Could you check a few things on this model? Use its own coordinates, in mm. A direction names the side the tool comes from. Round coordinates to 2 decimals unless told otherwise and drop trailing zeros. Order: outer loops, then holes, each group sorted by start corner. A loop starts at its lowest first (then second) coordinate and runs counter-clockwise, first axis right, second up. Notation, with made-up numbers: (-17.75, 71) -> (41.25, 71) arc R19 ccw to (41.25, 90) -> close; hole circle Ø9 at (2.25, 44.25). An arc over 180 degrees is marked (long way). Put each result on its own line as item: value. Start each with the question number.
from build123d import *

# Parameters (mm, degrees)
BOSS_EXTRUDE1_DEPTH            = 1.14
F_3_2_3_2_DIAMETER_HOLE1_D     = 3.2
F_3_2_3_2_DIAMETER_HOLE1_DEPTH = 10
F_3_2_3_2_DIAMETER_HOLE1_TIP   = 0.96137699


with BuildPart() as part:
    # Sketch1 → Boss-Extrude1 (new body, symmetric)
    with BuildSketch(Plane(origin=(0, 0, 2279.99997139), x_dir=(1, 0, 0), z_dir=(0, 1, 0))):
        with BuildLine():
            Line((10, 2292.262711431), (10, 2309.99997139))
            Line((10, 2309.99997139), (0, 2309.99997139))
            Line((0, 2309.99997139), (0, 2279.99997139))
            Line((0, 2279.99997139), (20, 2279.99997139))
            Line((20, 2279.99997139), (20, 2289.99997139))
            Line((20, 2289.99997139), (12.262740041, 2289.99997139))
            ThreePointArc((12.262740041, 2289.99997139), (9.99862915, 2289.99860054), (10, 2292.262711431))
        make_face()
    extrude(amount=BOSS_EXTRUDE1_DEPTH, both=True)

    # Ø3.2 (3.2) Diameter Hole1
    with Locations(Plane(origin=(0, 1.14, 0), x_dir=(1, 0, 0), z_dir=(0, 1, 0))):
        with Locations((5, 25), (5, 5), (15, 5), (5, 15)):
            Hole(F_3_2_3_2_DIAMETER_HOLE1_D / 2, depth=F_3_2_3_2_DIAMETER_HOLE1_DEPTH)
            with Locations((0, 0, -(F_3_2_3_2_DIAMETER_HOLE1_DEPTH + F_3_2_3_2_DIAMETER_HOLE1_TIP / 2))):  # 118° drill point
                Cone(0, F_3_2_3_2_DIAMETER_HOLE1_D / 2, F_3_2_3_2_DIAMETER_HOLE1_TIP, mode=Mode.SUBTRACT)


solid = part.part
1. Thinking about a two-plate mould opening in Z: for faces 1 (the face through (5, 0, -30)), 2 (the face through (16.6, -0.02, -5.07)), 3 (the face through (10, 0, -21)), which applies, +Z half, -Z half, draft (parallel to the pull), parting line (faces both ways), or undercut?
2. If we section it at A-A, the plane x = 5: Please give me the cut outline in (y, z), then the cut area to 3 significant figures.
3. If we section it at D-D, the plane x = 15: Please give me the cut outline in (y, z), then the cut area to 3 significant figures.
4. I need wall thicknesses on L1, parallel to Z at x = 5, y = -0.6; L2, parallel to X at y = 0.05, z = -5; L3, parallel to X at y = -0.2, z = -15. Which ranges of each line are inside material? Lowest first, please.
5. If we section it at B-B, the plane y = -0.2: Please give me the cut outline in (x, z), then the cut area to 3 significant figures.
6. For pin 1 Ø0.7 at (y, z) = (0.5, -17.5) entering from +X; pin 2 Ø1 at (x, y) = (12, 0.5) entering from -Z, each with a flat end and sliding along its axis, tell me the tip position at first contact or that it passes through.
7. Which directions (+Z, -Z, +X, -X, +Y, -Y) give clear straight access to the entire face, cutting with the end or side of a thin tool? Please do faces 4 (the face through (8, 1.14, -12)), 5 (the face through (16, 0, -10)).
8. If we section it at C-C, the plane z = -5: Please give me the cut outline in (x, y), then the cut area to 3 significant figures.
Results below:
1. face 1: -Z half
1. face 2: undercut
1. face 3: draft
2. outline: (-1.14, -30) -> (1.14, -30) -> (1.14, -26.6) -> (-1.14, -26.6) -> close; (-1.14, -23.4) -> (1.14, -23.4) -> (1.14, -16.6) -> (-1.14, -16.6) -> close; (-1.14, -13.4) -> (1.14, -13.4) -> (1.14, -6.6) -> (-1.14, -6.6) -> close; (-1.14, -3.4) -> (1.14, -3.4) -> (1.14, 0) -> (-1.14, 0) -> close
2. area: 46.5 mm2
3. outline: (-1.14, -10) -> (1.14, -10) -> (1.14, -6.6) -> (-1.14, -6.6) -> close; (-1.14, -3.4) -> (1.14, -3.4) -> (1.14, 0) -> (-1.14, 0) -> close
3. area: 15.5 mm2
4. L1: -30 to -26.6, -23.4 to -16.6, -13.4 to -6.6, -3.4 to 0
4. L2: 0 to 3.4, 6.6 to 13.4, 16.6 to 20
4. L3: 0 to 3.4, 6.6 to 10
5. outline: (0, -30) -> (10, -30) -> (10, -12.26) arc R1.6 cw to (12.26, -10) -> (20, -10) -> (20, 0) -> (0, 0) -> close; hole circle Ø3.2 at (5, -25); hole circle Ø3.2 at (5, -15); hole circle Ø3.2 at (5, -5); hole circle Ø3.2 at (15, -5)
5. area: 366 mm2
6. pin 1: x = 10
6. pin 2: z = -10
7. face 4: +Z, -Z, +X, -X, +Y
7. face 5: -Z, +X, +Y, -Y
8. outline: (0, -1.14) -> (3.4, -1.14) -> (3.4, 1.14) -> (0, 1.14) -> close; (6.6, -1.14) -> (13.4, -1.14) -> (13.4, 1.14) -> (6.6, 1.14) -> close; (16.6, -1.14) -> (20, -1.14) -> (20, 1.14) -> (16.6, 1.14) -> close
8. area: 31.0 mm2
